Read the model definition and answer for the solid it produces. Units are mm, in the model's axes. Face numbers are marked on the shaded views. A direction names the side the tool comes from. Give positions to 0.01 mm unless a question says otherwise; leave off trailing zeros. Loops run counter-clockwise (first coordinate to the right, second up) from the corner with the lowest first, then second, coordinate; pieces in that order, holes last.
(1) Find section B-B, the plane x = -16.5. Write down the section's boundary in (y, z), then the cut area to 3 significant figures.
(2) Find section D-D, the plane z = 8. Write down the section's boundary in (x, y).
(3) Find section A-A, the plane z = 0. Write down the section's boundary in (x, y), then the cut area to 3 significant figures.
(4) Straight lines are drawn through the part: probe 1 along X at (y, z) = (0.7, 0); probe 2 along Z at (x, y) = (0, -9.35); probe 3 along Z at (x, y) = (17.5, 0.25). For each, find the intervals that lie inside material, in ascending order.
(5) Which of the six approach directions +Z, -Z, +X, -X, +Y, -Y give full straight-line access (tool end or side, diameter ignored) to the marked faces 1, 2 and 3?
(6) Find section C-C, the plane y = 4.5. Write down the section's boundary in (x, z) (3 decimals), then the cut area to 3 significant figures.
(7) Each of these flat-tipped pins is pushed along its axis until it touches: P1, Ø0.8, axis at x = 2, z = 9, coming from the -Y side; P2, Ø5.5, axis at x = 18, z = 1, coming from the +Y side; P3, Ø1, axis at y = 6.5, z = -12, coming from the -X side (3 decimals). Where does it stop, or does it pass through?
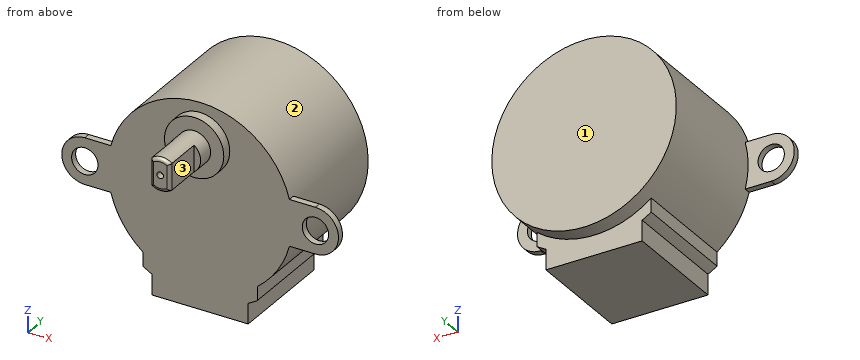
```python
from build123d import *

# Parameters (mm, degrees)
SKETCH1_R           = 14
BOSS_EXTRUDE1_DEPTH = 19
BOSS_EXTRUDE2_DEPTH = 16.5
SKETCH3_R           = 2
BOSS_EXTRUDE3_DEPTH = 1
SKETCH4_R           = 4.5
BOSS_EXTRUDE4_DEPTH = 1.5
SKETCH5_R           = 2.5
BOSS_EXTRUDE5_DEPTH = 2.5
BOSS_EXTRUDE6_DEPTH = 6
FILLET1_R           = 0.5
SKETCH7_R           = 0.5
CUT_EXTRUDE1_DEPTH  = 1


with BuildPart() as part:
    # Sketch1 → Boss-Extrude1 (new body)
    with BuildSketch(Plane(origin=(0, 0, 0), x_dir=(1, 0, 0), z_dir=(0, 1, 0))):
        Circle(SKETCH1_R)
    extrude(amount=BOSS_EXTRUDE1_DEPTH)

    # Sketch2 → Boss-Extrude2 (add)
    with BuildSketch(Plane(origin=(0, 0, 0), x_dir=(1, 0, 0), z_dir=(0, 1, 0))):
        with BuildLine():
            Line((7.3, 17), (-7.3, 17))
            Line((-7.3, 17), (-7.3, 13.902200296))
            ThreePointArc((-7.3, 13.902200296), (-7.99785811, 13.51278797), (-8.675, 13.088374539))
            Line((-8.675, 13.088374539), (-8.675, 10.988374539))
            ThreePointArc((-8.675, 10.988374539), (0, 14), (8.675, 10.988374539))
            Line((8.675, 10.988374539), (8.675, 13.088374539))
            ThreePointArc((8.675, 13.088374539), (7.99785811, 13.51278797), (7.3, 13.902200296))
            Line((7.3, 13.902200296), (7.3, 17))
        make_face()
    extrude(amount=BOSS_EXTRUDE2_DEPTH)

    # Sketch3 → Boss-Extrude3 (add)
    with BuildSketch(Plane(origin=(0, 0, 0), x_dir=(1, 0, 0), z_dir=(0, 1, 0))):
        with BuildLine():
            Line((-17.5, 3.5), (-13.555441712, 3.5))
            ThreePointArc((-13.555441712, 3.5), (-14, 0), (-13.555441712, -3.5))
            Line((-13.555441712, -3.5), (-17.5, -3.5))
            ThreePointArc((-17.5, -3.5), (-21, 0), (-17.5, 3.5))
        make_face()
        with Locations((-17.5, 0)):
            Circle(SKETCH3_R, mode=Mode.SUBTRACT)
        with BuildLine():
            Line((17.5, 3.5), (13.555441712, 3.5))
            ThreePointArc((13.555441712, 3.5), (14, 0), (13.555441712, -3.5))
            Line((13.555441712, -3.5), (17.5, -3.5))
            ThreePointArc((17.5, -3.5), (21, 0), (17.5, 3.5))
        make_face()
        with Locations((17.5, 0)):
            Circle(SKETCH3_R, mode=Mode.SUBTRACT)
    extrude(amount=BOSS_EXTRUDE3_DEPTH)

    # Sketch4 → Boss-Extrude4 (add)
    with BuildSketch(Plane.XZ):
        with Locations((0, 8)):
            Circle(SKETCH4_R)
    extrude(amount=BOSS_EXTRUDE4_DEPTH)

    # Sketch5 → Boss-Extrude5 (add)
    with BuildSketch(Plane.XZ.offset(1.5)):
        with Locations((0, 8)):
            Circle(SKETCH5_R)
    extrude(amount=BOSS_EXTRUDE5_DEPTH)

    # Sketch6 → Boss-Extrude6 (add)
    with BuildSketch(Plane.XZ.offset(4)):
        with BuildLine():
            Line((-1.5, 10), (-1.5, 6))
            ThreePointArc((-1.5, 6), (0, 5.5), (1.5, 6))
            Line((1.5, 6), (1.5, 10))
            ThreePointArc((1.5, 10), (0, 10.5), (-1.5, 10))
        make_face()
    extrude(amount=BOSS_EXTRUDE6_DEPTH)

    # Fillet1
    fillet1_edges = [part.edges().sort_by_distance(p)[0] for p in [
        (0, -10, 10.5),
        (-1.5, -10, 8),
        (0, -10, 5.5),
        (1.5, -10, 8),
    ]]
    fillet(fillet1_edges, radius=FILLET1_R)

    # Sketch7 → Cut-Extrude1 (cut)
    with BuildSketch(Plane.XZ.offset(10)):
        with Locations((0, 8)):
            Circle(SKETCH7_R)
    extrude(amount=-CUT_EXTRUDE1_DEPTH, mode=Mode.SUBTRACT)


solid = part.part
```
Entries:
1. outline: (0, -3.5) - (1, -3.5) - (1, -1.73) - (0, -1.73) - close; (0, 1.73) - (1, 1.73) - (1, 3.5) - (0, 3.5) - close
1. area: 3.54 mm2
2. outline: (-11.49, 0) - (-4.5, 0) - (-4.5, -1.5) - (-2.5, -1.5) - (-2.5, -4) - (-1.5, -4) - (-1.5, -9.5) arc R0.5 ccw to (-1, -10) - (-0.5, -10) - (-0.5, -9) - (0.5, -9) - (0.5, -10) - (1, -10) arc R0.5 ccw to (1.5, -9.5) - (1.5, -4) - (2.5, -4) - (2.5, -1.5) - (4.5, -1.5) - (4.5, 0) - (11.49, 0) - (11.49, 19) - (-11.49, 19) - close
3. outline: (-21, 0) - (-19.5, 0) - (-19.5, 1) - (-21, 1) - close; (-15.5, 0) - (15.5, 0) - (15.5, 1) - (14, 1) - (14, 19) - (-14, 19) - (-14, 1) - (-15.5, 1) - close; (19.5, 0) - (21, 0) - (21, 1) - (19.5, 1) - close
3. area: 538 mm2
4. probe 1: x = -21 to -19.5, -15.5 to 15.5, 19.5 to 21
4. probe 2: z = 5.5 to 7.5, 8.5 to 10.5
4. probe 3: z = -3.5 to -2, 2 to 3.5
5. face 1: +Z, -Z, +X, -X, +Y
5. face 2: +Y
5. face 3: +Z, -Z, +X, -Y
6. outline: (-8.675, -13.088) arc R15.702 ccw to (-7.3, -13.902) - (-7.3, -17) - (7.3, -17) - (7.3, -13.902) arc R15.702 ccw to (8.675, -13.088) - (8.675, -10.988) arc R14 ccw (long way) to (-8.675, -10.988) - close
6. area: 675 mm2
7. P1: stops at y = -4
7. P2: stops at y = 1
7. P3: stops at x = -8.675
